from build123d import *

# Parameters (mm, degrees)
F0_R     = 12.7
F0_W     = 44.1198
F0_H     = 22.352
F0_W_2   = 32.8422
F1_DEPTH = 60.325
F2_DEPTH = 19.05
F3_W     = 33.1412
F3_H     = 22.3266
F3_W_2   = 55.289626
F3_R     = 6.35
F4_DEPTH = 57.151
F6_DEPTH = 41.275
F7_R     = 5.08
F8_R     = 7.62


with BuildPart() as f1:
    # F0 (on Front) → F1 (new body)
    with BuildSketch(Plane.XZ):
        with BuildLine():
            ThreePointArc((22.352, 0), (0, 22.352), (-22.352, 0))
            ThreePointArc((-22.352, 0), (-15.805251, -15.805251), (0, -22.352))
            Line((0, -22.352), (91.8464, -22.352))
            Line((91.8464, -22.352), (85.852, 0))
            Line((85.852, 0), (22.352, 0))
        make_face()
        Circle(F0_R, mode=Mode.SUBTRACT)
        Polygon((85.852, 0), (91.8464, -22.352), (117.2464, -22.352), (117.2464, 0), align=None)
        with Locations((172.1485, -11.176)):
            Rectangle(F0_W, F0_H)
        with BuildLine():
            ThreePointArc((131.0386, 34.798), (127.464415, 16.082358), (117.2464, 0))
            Line((117.2464, 0), (150.0886, 0))
            Line((150.0886, 0), (150.0886, 34.798))
            Line((150.0886, 34.798), (131.0386, 34.798))
        make_face()
        with Locations((133.6675, -11.176)):
            Rectangle(F0_W_2, F0_H)
    extrude(amount=-F1_DEPTH)

    # F0 (on Front) → F2 (cut)
    with BuildSketch(Plane.XZ):
        Polygon((85.852, 0), (91.8464, -22.352), (117.2464, -22.352), (117.2464, 0), align=None)
    extrude(amount=-F2_DEPTH, mode=Mode.SUBTRACT)

    # F3 (on face) → F4 (cut, through all)
    with BuildSketch(Plane(origin=(0, 0, -22.352), x_dir=(1, 0, 0), z_dir=(0, 0, -1))):
        with Locations((16.5706, -30.1625)):
            Rectangle(F3_W, F3_H)
        with Locations((-27.644813, -30.1625)):
            Rectangle(F3_W_2, F3_H)
        with Locations((155.3464, -37.973)):
            Circle(F3_R)
    extrude(amount=-F4_DEPTH, mode=Mode.SUBTRACT)

    # F5 (on face) → F6 (cut)
    with BuildSketch(Plane(origin=(0, 60.325, 0), x_dir=(-1, 0, 0), z_dir=(0, 1, 0))):
        with BuildLine():
            Line((-150.0886, 0), (-117.2464, 0))
            ThreePointArc((-117.2464, 0), (-127.464415, 16.082358), (-131.0386, 34.798))
            Line((-131.0386, 34.798), (-150.0886, 34.798))
            Line((-150.0886, 34.798), (-150.0886, 0))
        make_face()
    extrude(amount=-F6_DEPTH, mode=Mode.SUBTRACT)

    # F7
    f7_edges = [f1.edges().sort_by_distance(p)[0] for p in [
        (22.352, 9.4996, 0),
        (22.352, 50.8254, 0),
        (150.0886, 9.525, 34.798),
        (150.0886, 9.525, 0),
    ]]
    fillet(f7_edges, radius=F7_R)

    # F8
    f8_edges = [f1.edges().sort_by_distance(p)[0] for p in [
        (194.2084, 30.1625, 0),
    ]]
    fillet(f8_edges, radius=F8_R)


solid = f1.part
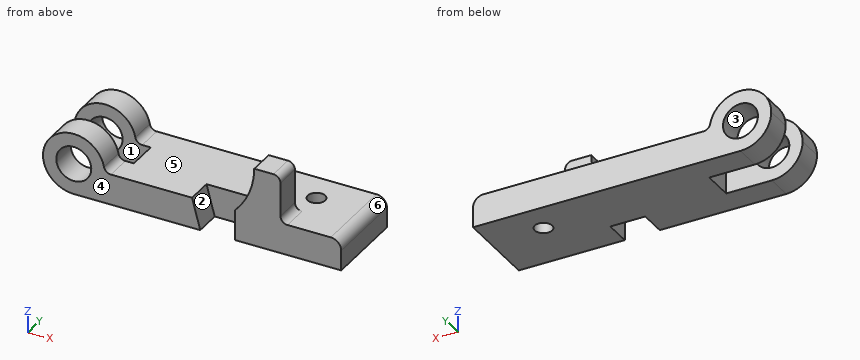
CAD build for the part. Positions are in the model's coordinates, mm. Face numbers are marked on the shaded views. A direction names the side the tool comes from. Round coordinates to 2 decimals unless told otherwise and drop trailing zeros. Loops run counter-clockwise (first coordinate to the right, second up) from the corner with the lowest first, then second, coordinate; pieces in that order, holes last.
(1) Two-plate mould, pull along X, no slides. Class the marked faces 4, 5 and 6: +X half, -X half, draft (parallel to the pull), parting line (faces both ways), or undercut.
(2) Cut at C-C (z = 10.5). Give the cut face in (x, y) (3 decimals), plus the area to 3 significant figures.
(3) Which spindle directions (+Z, -Z, +X, -X, +Y, -Y) get a long thin tool onto all of the face, cutting with end or side? Do the marked faces 1, 2 and 3. Say none if no direction does.
(4) Cut at A-A (y = 4). Give the cut face in (x, z), plus the area to 3 significant figures.
(5) Wall check: line 1 along Y through (x, z) = (31.5, -0.5) (3 decimals); line 2 along Z through (x, y) = (51, 6); line 3 along X through (y, z) = (39, -6). Give the ranges that are in metal, low to high.
(6) Drop flat-ended pins along their axis: pin 1 (7.5 mm diameter, centred on x = 155.35, y = 37.97, fed in from +Z); pin 2 (8 mm diameter, centred on x = 31, y = 50.5, fed in from +Z); pin 3 (6.5 mm diameter, centred on y = 34, z = -14, fed in from -X); pin 4 (17.5 mm diameter, centred on x = 145, z = 23.5, fed in from +Y). Give the stop position or say it passes through.
(7) Cut at B-B (y = 53.5). Give the cut face in (x, z).
(8) Cut at D-D (x = 138.5). Give the cut face in (y, z) (3 decimals), plus the area to 3 significant figures.
Findings below:
1. face 4: draft
1. face 5: undercut
1. face 6: +X half
2. outline: (-19.732, 0) - (-7.144, 0) - (-7.144, 18.999) - (-19.732, 18.999) - close; (-19.732, 41.326) - (-7.144, 41.326) - (-7.144, 60.325) - (-19.732, 60.325) - close; (7.144, 0) - (19.732, 0) - (19.732, 18.999) - (7.144, 18.999) - close; (7.144, 41.326) - (19.732, 41.326) - (19.732, 60.325) - (7.144, 60.325) - close; (124.85, 0) - (150.089, 0) - (150.089, 19.05) - (124.85, 19.05) - close
2. area: 1,440 mm2
3. face 1: +Z, -Z, -X
3. face 2: +Z, -Y
3. face 3: +Y, -Y
4. outline: (0, -22.35) - (91.85, -22.35) - (85.85, 0) - (26.96, 0) arc R5.08 cw to (21.97, 4.14) arc R22.35 ccw (long way) to start; (117.25, -22.35) - (194.21, -22.35) - (194.21, -7.62) arc R7.62 ccw to (186.59, 0) - (155.17, 0) arc R5.08 cw to (150.09, 5.08) - (150.09, 29.72) arc R5.08 ccw to (145.01, 34.8) - (131.04, 34.8) arc R50.8 cw to (117.25, 0) - close; hole circle Ø25.4 at (0, 0)
4. area: 5,180 mm2
5. line 1: y = 0 to 18.999, 41.326 to 60.325
5. line 2: z = -22.35 to 0
5. line 3: x = 33.14 to 149.08, 161.61 to 194.03
6. pin 1: passes through
6. pin 2: stops at z = 0
6. pin 3: stops at x = 33.14
6. pin 4: stops at y = 19.05
7. outline: (0, -22.35) - (194.21, -22.35) - (194.21, -7.62) arc R7.62 ccw to (186.59, 0) - (26.96, 0) arc R5.08 cw to (21.97, 4.14) arc R22.35 ccw (long way) to start; hole circle Ø25.4 at (0, 0)
8. outline: (0, -22.352) - (60.325, -22.352) - (60.325, 0) - (19.05, 0) - (19.05, 34.798) - (0, 34.798) - close
8. area: 2,010 mm2
